```python
from build123d import *

# Parameters (mm, degrees)
SKETCH_1_R          = 65
EXTRUDE_1_DEPTH     = 3
SKETCH_2_R          = 2
SKETCH_2_R_2        = 1.5
CUT_EXTRUDE_4_DEPTH = 3


with BuildPart() as part:
    # 草图1 → 凸台-拉伸1 (new body)
    with BuildSketch(Plane.XY):
        Circle(SKETCH_1_R)
    extrude(amount=EXTRUDE_1_DEPTH)

    # 草图2 → 切除-拉伸4 (cut)
    with BuildSketch(Plane.XY.offset(3)):
        with Locations((40, 0)):
            Circle(SKETCH_2_R)
        with Locations((50, -10)):
            Circle(SKETCH_2_R)
        with Locations((50, 0)):
            Circle(SKETCH_2_R_2)
        with Locations((50, 0)):
            Circle(SKETCH_2_R)
        with Locations((50, 10)):
            Circle(SKETCH_2_R)
        with Locations((60, 0)):
            Circle(SKETCH_2_R)
    extrude(amount=-CUT_EXTRUDE_4_DEPTH, mode=Mode.SUBTRACT)


solid = part.part
```
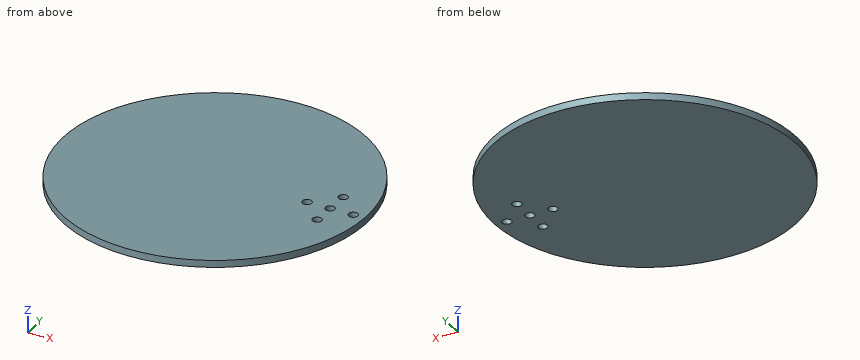
Build history of the part. All positions in model axes, mm. Give positions to 0.01 mm unless a question says otherwise; leave off trailing zeros. Order: outer loops, then holes, each group sorted by start corner. A loop starts at its lowest first (then second) coordinate and runs counter-clockwise, first axis right, second up. Notation, with made-up numbers: M 0.5,36.25 L 5.5,36.25 A7 cw 5.5,49.25 Z; hole C 22,36.25 d5. An arc over 180 degrees is marked long. Return JSON: item names as keys, results as strings.
Q1. Band-saw the part on A-A (y = 0). Give the cut face in (x, z).
Answer list:
{"outline": "M -65,0 L 38,0 L 38,3 L -65,3 Z; M 42,0 L 48,0 L 48,3 L 42,3 Z; M 52,0 L 58,0 L 58,3 L 52,3 Z; M 62,0 L 65,0 L 65,3 L 62,3 Z"}
Q2. Band-saw the part on D-D (x = 40). Give the cut face in (y, z), then the cut area to 3 significant figures.
Answer list:
{"outline": "M -51.23,0 L -2,0 L -2,3 L -51.23,3 Z; M 2,0 L 51.23,0 L 51.23,3 L 2,3 Z", "area": "295 mm^2"}
Q3. Band-saw the part on C-C (z = 0.75). Give the cut face in (x, y), then the cut area to 3 significant figures.
Answer list:
{"outline": "C 0,0 d130; hole C 40,0 d4; hole C 50,-10 d4; hole C 50,0 d4; hole C 50,10 d4; hole C 60,0 d4", "area": "13,200 mm^2"}
Q4. Flat gauge pins, fed straight in: pin 1 (5 mm diameter, centred on x = 7, y = 25.5, fed in from -Z); pin 2 (3.5 mm diameter, centred on x = 50, y = -10, fed in from -Z); pin 3 (1.5 mm diameter, centred on x = 12, z = 1, fed in from +Y). Where does each tip first touch, or does it go through?
Answer list:
{"pin 1": "stops at z = 0", "pin 2": "passes through", "pin 3": "stops at y = 64.02"}
Q5. Band-saw the part on B-B (x = 60). Give the cut face in (y, z).
Answer list:
{"outline": "M -25,0 L -2,0 L -2,3 L -25,3 Z; M 2,0 L 25,0 L 25,3 L 2,3 Z"}
Q6. Wall check: probe 1 along Y at (x, z) = (50, 1.75); probe 2 along Y at (x, z) = (0.5, 1.15); probe 3 along Y at (x, z) = (-45.5, 1.2). Give the ranges that are in metal, low to high. Write a range as from..to.
Answer list:
{"probe 1": "y = -41.53..-12, -8..-2, 2..8, 12..41.53", "probe 2": "y = -65..65", "probe 3": "y = -46.42..46.42"}
